The model under review builds one solid part; all positions refer to its coordinate system, in mm. Face numbers are marked on the shaded views. A direction names the side the tool comes from. Round coordinates to 2 decimals unless told otherwise and drop trailing zeros. Order: outer loops, then holes, each group sorted by start corner. A loop starts at its lowest first (then second) coordinate and runs counter-clockwise, first axis right, second up.
1) Consider section D-D (x = 24.5). Give the boundary of the cut face in (y, z), then the cut area to 3 significant figures.
2) Machinability: for the marked faces 1, 2, 3 and 4, which of the approach directions +Z, -Z, +X, -X, +Y, -Y give a long, thin tool a straight path to every point of the face, cutting with its end or side? Answer none if there is none.
3) Mouldability with a two-part tool opening along X and no side actions: class the marked faces 5, 6 and 7 as pulls with the +X half, pulls with the -X half, needs draft (parallel to the pull), parting line crosses it, or undercut.
4) Consider section B-B (x = 20). Give the boundary of the cut face in (y, z), then the cut area to 3 significant figures.
5) Consider section C-C (z = 1.5). Give the number of separate pieces and of enclosed holes in the cut face, then the cut area to 3 significant figures.
6) Clearance check with flat-ended pins moving along their axes: P1, Ø3.5, axis at x = 19.62, y = 0.95, coming from the -Z side; P2, Ø3, axis at y = 4, z = -1, coming from the -X side; P3, Ø2, axis at y = 11, z = 2.5, coming from the +X side; P4, Ø0.9, axis at x = 1.5, y = 1, coming from the +Z side. State where each tip first meets the part, or that it passes through.
7) To check wall thickness, follow L1, parallel to X at y = 1, z = 3.5; L2, parallel to Z at x = 10, y = 18; L3, parallel to X at y = 2, z = -2. State the ranges of each line that lie inside material, in increasing order.
8) Consider section A-A (y = -1.5). Give the boundary of the cut face in (x, z), then the cut area to 3 significant figures.
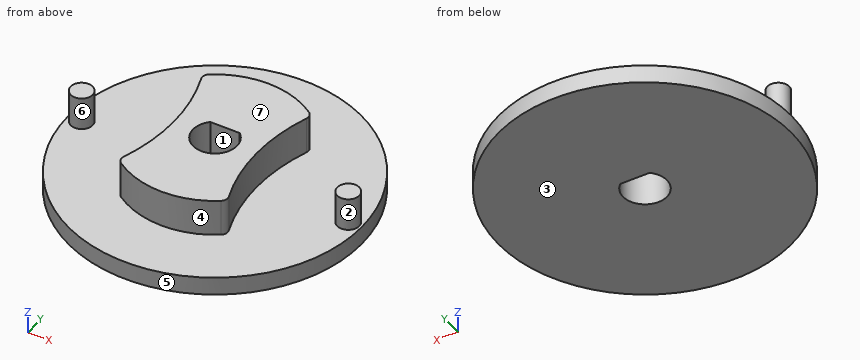
from build123d import *

# Parameters (mm, degrees)
BOSS_EXTRUDE1_DEPTH     = 5
SKETCH2_R               = 20
BOSS_EXTRUDE2_DEPTH     = 2.5
SKETCH3_R               = 1.5
BOSS_EXTRUDE3_DEPTH     = 4.5
CUT_EXTRUDE1_DEPTH      = 6
CUT_EXTRUDE1_DEPTH_BACK = 3.5
FILLET1_R               = 1


with BuildPart() as part:
    # Sketch1 → Boss-Extrude1 (new body)
    with BuildSketch(Plane.XY):
        with BuildLine():
            ThreePointArc((27.055367122, -8.375602421), (25.270767556, 0.948424737), (27.055367122, 10.272451896))
            ThreePointArc((27.055367122, 10.272451896), (19.619068119, 12.874699316), (12.182769116, 10.272451896))
            ThreePointArc((12.182769116, 10.272451896), (13.967368681, 0.948424737), (12.182769116, -8.375602421))
            ThreePointArc((12.182769116, -8.375602421), (19.619068119, -10.977849841), (27.055367122, -8.375602421))
        make_face()
    extrude(amount=BOSS_EXTRUDE1_DEPTH)

    # Sketch2 → Boss-Extrude2 (add)
    with BuildSketch(Plane.XY):
        with Locations((19.619068119, 0.948424737)):
            Circle(SKETCH2_R)
    extrude(amount=-BOSS_EXTRUDE2_DEPTH)

    # Sketch3 → Boss-Extrude3 (add)
    with BuildSketch(Plane.XY):
        with Locations((1.455504919, 0.948424737)):
            Circle(SKETCH3_R)
        with Locations((37.782631319, 0.948424737)):
            Circle(SKETCH3_R)
    extrude(amount=BOSS_EXTRUDE3_DEPTH)

    # Sketch4 → Cut-Extrude1 (cut, two sides)
    with BuildSketch(Plane.XY) as cut_extrude1_sk:
        with BuildLine():
            Line((17.619068119, 3.184492715), (21.619068119, 3.184492715))
            ThreePointArc((21.619068119, 3.184492715), (19.619068119, -2.051575263), (17.619068119, 3.184492715))
        make_face()
    extrude(amount=CUT_EXTRUDE1_DEPTH, mode=Mode.SUBTRACT)
    extrude(cut_extrude1_sk.sketch, amount=-CUT_EXTRUDE1_DEPTH_BACK, mode=Mode.SUBTRACT)

    # Fillet1
    fillet1_edges = [part.edges().sort_by_distance(p)[0] for p in [
        (12.182769116, -8.375602421, 2.5),
        (12.182769116, 10.272451896, 2.5),
        (27.055367122, 10.272451896, 2.5),
        (27.055367122, -8.375602421, 2.5),
    ]]
    fillet(fillet1_edges, radius=FILLET1_R)


solid = part.part
Answer below:
1. outline: (-18.45, -2.5) - (20.34, -2.5) - (20.34, 0) - (11.83, 0) - (11.83, 5) - (-9.93, 5) - (-9.93, 0) - (-18.45, 0) - close
1. area: 206 mm2
2. face 1: +Z, -Z
2. face 2: +Z
2. face 3: -Z, +X, -X, +Y, -Y
2. face 4: +Z, -Y
3. face 5: parting line crosses it
3. face 6: undercut
3. face 7: needs draft
4. outline: (-19.05, -2.5) - (-2.03, -2.5) - (-2.03, 5) - (-10.97, 5) - (-10.97, 0) - (-19.05, 0) - close; (3.18, -2.5) - (20.94, -2.5) - (20.94, 0) - (12.87, 0) - (12.87, 5) - (3.18, 5) - close
4. area: 180 mm2
5. separate pieces: 3
5. enclosed holes: 1
5. area: 273 mm2
6. P1: passes through
6. P2: stops at x = -0.32
6. P3: stops at x = 26.85
6. P4: stops at z = 4.5
7. L1: x = -0.04 to 2.95, 13.97 to 16.62, 22.62 to 25.27, 36.28 to 39.28
7. L2: z = -2.5 to 0
7. L3: x = -0.35 to 16.81, 22.43 to 39.59
8. outline: (-0.23, -2.5) - (17.89, -2.5) - (17.89, 5) - (13.85, 5) - (13.85, 0) - (-0.23, 0) - close; (21.35, -2.5) - (39.47, -2.5) - (39.47, 0) - (25.39, 0) - (25.39, 5) - (21.35, 5) - close
8. area: 131 mm2
